For this review, use the dimensioned drawing (mm, ordinates from the lowest corner) and the shaded views. Coordinates: 2 decimals unless noted, no trailing zeros. Write each loop counter-clockwise with the first axis right and the second up, starting at its lowest first coordinate (ties: lowest second). Pieces come first, ordered by that corner, then holes. Notation, with made-up numbers: (-1.5, 65.5) - (33.5, 65.5) arc R19 ccw to (33.5, 85.5) - close; hole circle Ø10 at (80, 55.5). An arc over 180 degrees is marked (long way). Answer as a JSON object with one key per item and string values.
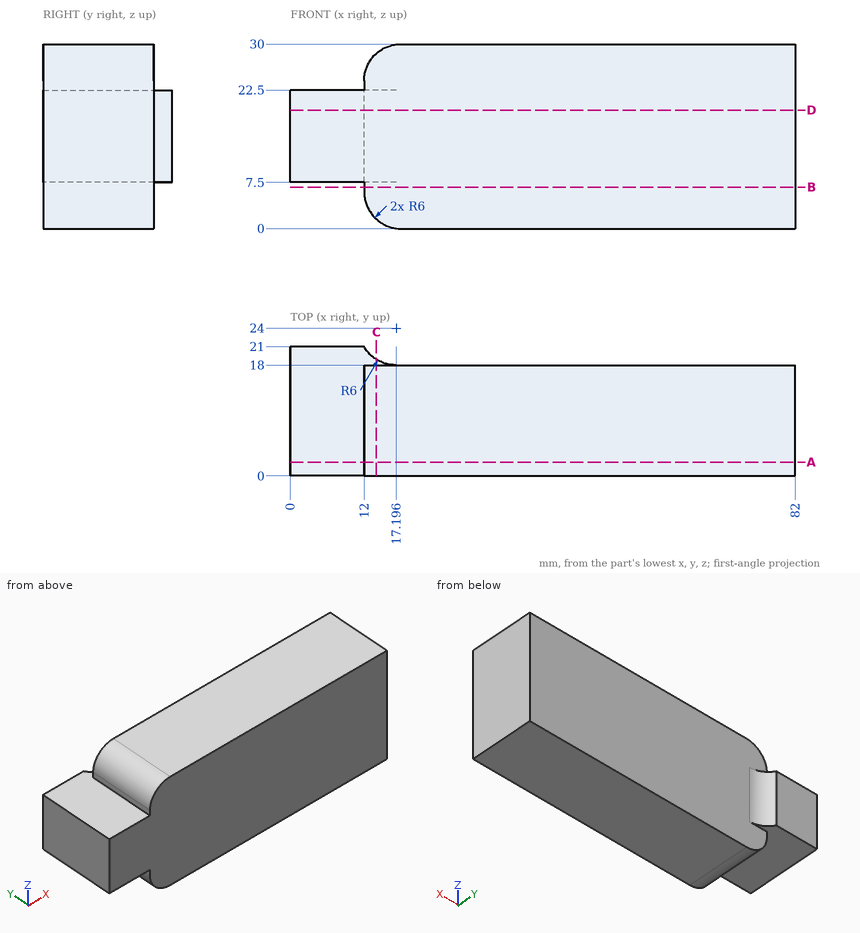
(1) Take a section at D-D, the plane z = 19.25. Write out the cut boundary in (x, y), and give its area (3 significant figures).
Solved:
{"outline": "(0, 0) - (82, 0) - (82, 18) - (17.2, 18) arc R6 cw to (12, 21) - (0, 21) - close", "area": "1,520 mm^2"}
(2) Take a section at C-C, the plane x = 14. Write out the cut boundary in (y, z), and give its area (3 significant figures).
Solved:
{"outline": "(0, 1.53) - (18, 1.53) - (18, 7.5) - (18.92, 7.5) - (18.92, 22.5) - (18, 22.5) - (18, 28.47) - (0, 28.47) - close", "area": "499 mm^2"}
(3) To check wall thickness, follow line 1 (Y direction, x = 46.5, z = 18.25); line 2 (X direction, y = 15.5, z = 23); line 3 (X direction, y = 8.5, z = 26.5). State the ranges of each line that lie inside material, in increasing order. Write a range as from..to.
Solved:
{"line 1": "y = 0..18", "line 2": "x = 12..82", "line 3": "x = 12.55..82"}
(4) Take a section at B-B, the plane z = 6.75. Write out the cut boundary in (x, y), and give its area (3 significant figures).
Solved:
{"outline": "(12, 0) - (82, 0) - (82, 18) - (12, 18) - close", "area": "1,260 mm^2"}
(5) Take a section at A-A, the plane y = 2.25. Write out the cut boundary in (x, z), and give its area (3 significant figures).
Solved:
{"outline": "(0, 7.5) - (12, 7.5) - (12, 6) arc R6 ccw to (18, 0) - (82, 0) - (82, 30) - (18, 30) arc R6 ccw to (12, 24) - (12, 22.5) - (0, 22.5) - close", "area": "2,260 mm^2"}
(6) For pin 1 (5 mm diameter, centred on x = 45, z = 17.5, fed in from +Y); pin 2 (1.6 mm diameter, centred on y = 6, z = 6.5, fed in from -X); pin 3 (8.5 mm diameter, centred on x = 10, y = 15.5, fed in from -Z), all flat-tipped, find the tip position at first contact; note any pin that passes through.
Solved:
{"pin 1": "stops at y = 18", "pin 2": "stops at x = 12", "pin 3": "stops at z = 1.32"}
